Check sheet for the drawn part. Datum: minimum x, y, z corner. Units: mm. A direction names the side the tool comes from. Give positions to 0.01 mm unless a question says otherwise; leave off trailing zeros. Order: outer loops, then holes, each group sorted by start corner. A loop starts at its lowest first (then second) coordinate and runs counter-clockwise, first axis right, second up. Notation, with made-up numbers: (-1, 1) - (53, 1) arc R25 cw to (53, 13) - close; hole circle Ø2 at (-3, 18). An arc over 180 degrees is marked (long way). Answer as a JSON object with one key per item and string values. Group by question number.
(1) Section check A-A (y = 4.5). Record the boundary of the cut face in (x, z), then the cut area to 3 significant figures.
(2) Thickness scan on line 1 (Y direction, x = 36.5, z = 0.6); line 2 (X direction, y = 10.5, z = 1.3); line 3 (X direction, y = 6.25, z = 4.45). Record the ranges inside material, lowest first.
(3) Section check C-C (x = 36.5). Record the boundary of the cut face in (y, z).
(4) Access from +Z, -Z, +X, -X, +Y, -Y to the whole of each face (thin tool, end or side, straight path). Record for the marked faces 4 and 5.
(5) Mould release check, pull along Y, two halves, no side actions. Record for the marked faces 1, 2 and 3: +Y half, -Y half, draft (parallel to the pull), parting line (faces both ways), or undercut.
(6) Section check B-B (z = 4.8). Record the boundary of the cut face in (x, y).
(7) Section check D-D (z = 2.3). Count the separate pieces of the cut face and the enclosed holes in it, then the cut area to 3 significant figures.
(8) Depth check by flat-ended pin: pin 1 Ø2 at (x, z) = (9.5, 2.5) entering from +Y; pin 2 Ø6 at (x, y) = (48, 5.5) entering from -Z; pin 3 Ø5 at (x, y) = (36.5, 10.5) entering from +Z. Enter the tip coordinate at first touch or a pass-through.
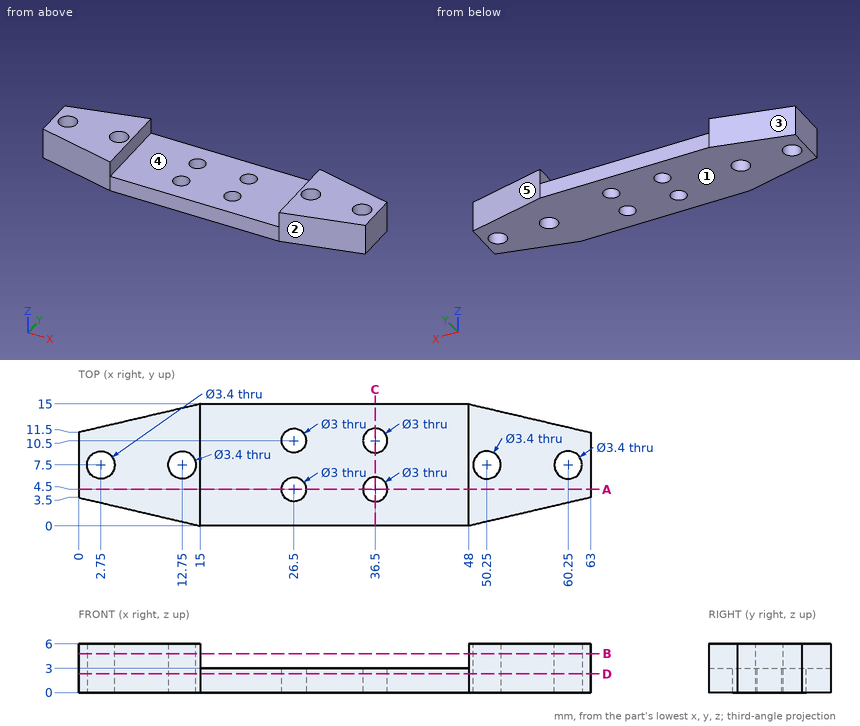
Solutions:
{
 "1": {"outline": "(0, 0) - (25, 0) - (25, 3) - (15, 3) - (15, 6) - (0, 6) - close; (28, 0) - (35, 0) - (35, 3) - (28, 3) - close; (38, 0) - (63, 0) - (63, 6) - (48, 6) - (48, 3) - (38, 3) - close", "area": "261 mm2"},
 "2": {"line 1": "y = 0 to 3, 6 to 9, 12 to 15", "line 2": "x = 0 to 25, 28 to 35, 38 to 63", "line 3": "x = 0 to 1.6, 3.9 to 11.6, 13.9 to 15, 48 to 49.1, 51.4 to 59.1, 61.4 to 63"},
 "3": {"outline": "(0, 0) - (3, 0) - (3, 3) - (0, 3) - close; (6, 0) - (9, 0) - (9, 3) - (6, 3) - close; (12, 0) - (15, 0) - (15, 3) - (12, 3) - close"},
 "4": {"face 4": "+Z, +Y, -Y", "face 5": "+Z, -Z, +X, +Y"},
 "5": {"face 1": "draft", "face 2": "-Y half", "face 3": "+Y half"},
 "6": {"outline": "(0, 3.5) - (15, 0) - (15, 15) - (0, 11.5) - close; (48, 0) - (63, 3.5) - (63, 11.5) - (48, 15) - close; hole circle Ø3.4 at (2.75, 7.5); hole circle Ø3.4 at (12.75, 7.5); hole circle Ø3.4 at (50.25, 7.5); hole circle Ø3.4 at (60.25, 7.5)"},
 "7": {"separate pieces": "1", "enclosed holes": "8", "area": "775 mm2"},
 "8": {"pin 1": "stops at y = 13.95", "pin 2": "stops at z = 0", "pin 3": "stops at z = 3"}
}
